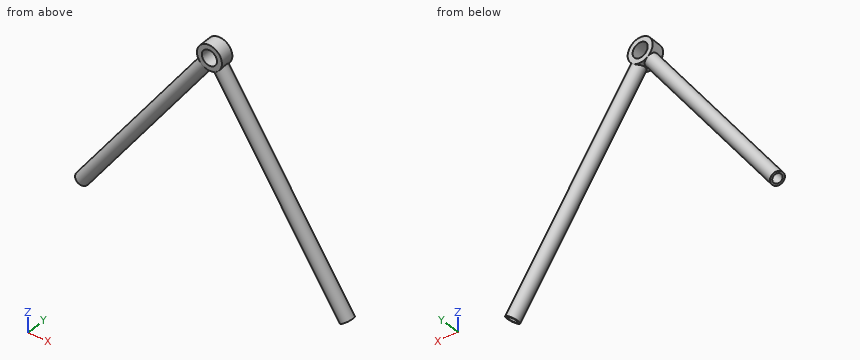
from build123d import *

# Parameters (mm, degrees)
SKETCH1_R                = 19.0062
SKETCH1_R_2              = 11.5062
BOSS_EXTRUDE1_DEPTH      = 10
BOSS_EXTRUDE2_REACH      = 392.082
BOSS_EXTRUDE2_END_RADIUS = 19.0062
SKETCH5_R                = 10
SKETCH5_R_2              = 7
BOSS_EXTRUDE3_REACH      = 510.057
BOSS_EXTRUDE3_END_RADIUS = 19.0062
SKETCH6_R                = 10
SKETCH6_R_2              = 7


with BuildPart() as part:
    # Sketch1 → Boss-Extrude1 (new, symmetric)
    with BuildSketch(Plane(origin=(0, 0, 0), x_dir=(1, 0, 0), z_dir=(0, 1, 0))):
        with Locations(Location((0, 0, 0), (0, 0, 270))):
            Circle(SKETCH1_R)
        with Locations(Location((0, 0, 0), (0, 0, 270))):
            Circle(SKETCH1_R_2, mode=Mode.SUBTRACT)
    extrude(amount=BOSS_EXTRUDE1_DEPTH, both=True)

    # Boss-Extrude2: up to this cylinder (the profile starts outside it)
    boss_extrude2_end = Plane(origin=(0, 0, 0), z_dir=(0, -1, 0)) * Cylinder(BOSS_EXTRUDE2_END_RADIUS, 823.1764, mode=Mode.PRIVATE)
    # Sketch5 → Boss-Extrude2 (add, up to the surface)
    with BuildSketch(Plane(origin=(201.884851726, 0, -302.352155823), x_dir=(0.8316479627965052, 0, 0.555303219850581), z_dir=(0.555303219850581, 0, -0.8316479627965052)), mode=Mode.PRIVATE) as boss_extrude2_sk1:
        with Locations(Location((0, 0, 0), (0, 0, 180))):
            Circle(SKETCH5_R)
        with Locations(Location((0, 0, 0), (0, 0, 180))):
            Circle(SKETCH5_R_2, mode=Mode.SUBTRACT)
    boss_extrude2_tool1 = extrude(boss_extrude2_sk1.sketch, amount=-BOSS_EXTRUDE2_REACH, mode=Mode.PRIVATE) - boss_extrude2_end
    add(boss_extrude2_tool1.solids().sort_by_distance((209.966106, 0, -296.956187))[0])

    # Boss-Extrude3: up to this cylinder (the profile starts outside it)
    boss_extrude3_end = Plane(origin=(0, 0, 0), z_dir=(0, -1, 0)) * Cylinder(BOSS_EXTRUDE3_END_RADIUS, 1059.1264, mode=Mode.PRIVATE)
    # Sketch6 → Boss-Extrude3 (add, up to the surface)
    with BuildSketch(Plane(origin=(-200.97050419, 0, -279.254437795), x_dir=(-0.811662071535183, 0, 0.5841272820466578), z_dir=(-0.5841272820466578, 0, -0.811662071535183)), mode=Mode.PRIVATE) as boss_extrude3_sk1:
        Circle(SKETCH6_R)
        Circle(SKETCH6_R_2, mode=Mode.SUBTRACT)
    boss_extrude3_tool1 = extrude(boss_extrude3_sk1.sketch, amount=-BOSS_EXTRUDE3_REACH, mode=Mode.PRIVATE) - boss_extrude3_end
    add(boss_extrude3_tool1.solids().sort_by_distance((-193.083456, 0, -284.930494))[0])


solid = part.part
For this review, take the finished solid that the model builds, in its own axes (mm). Give positions to 0.01 mm unless a question says otherwise; leave off trailing zeros. Order: outer loops, then holes, each group sorted by start corner. A loop starts at its lowest first (then second) coordinate and runs counter-clockwise, first axis right, second up. Notation, with made-up numbers: (-6, 7.25) -> (44, 7.25) arc R8 cw to (44, 12.25) -> close; hole circle Ø3 at (77, 61). An arc over 180 degrees is marked (long way). Write item = value, one per line.
1) We need section B-B, the plane y = 3.25. Give the boundary of the cut face in (x, z), and give its area (3 significant figures).
Findings:
outline = (-208.65, -273.73) -> (-206, -275.63) -> (-15.53, -10.96) arc R19.01 ccw to (-5.46, -18.2) -> (-195.94, -282.88) -> (-193.29, -284.78) -> (-1.95, -18.91) arc R19.01 ccw to (1.29, -18.96) -> (194.02, -307.6) -> (196.73, -305.79) -> (4.82, -18.38) arc R19.01 ccw to (15.13, -11.5) -> (207.04, -298.91) -> (209.75, -297.1) -> (17.02, -8.46) arc R19.01 ccw (long way) to (-17.31, -7.86) -> close; hole circle Ø23.01 at (0, 0)
area = 5,100 mm^2
2) We need section A-A, the plane z = 0. Give the boundary of the cut face in (x, y), and give its area (3 significant figures).
Findings:
outline = (-19.01, -10) -> (-11.51, -10) -> (-11.51, 10) -> (-19.01, 10) -> close; (11.51, -10) -> (19.01, -10) -> (19.01, 10) -> (11.51, 10) -> close
area = 300 mm^2
3) To check wall thickness, follow L1, parallel to X at y = 4.5, z = 0; L2, parallel to Y at x = 35.5, z = -52.5; L3, parallel to X at y = 1, z = -129. State the ranges of each line that lie inside material, in increasing order. Write a range as from..to.
Findings:
L1 = -19.01..-11.51, 11.51..19.01
L2 = -9.99..-6.99, 6.99..9.99
L3 = -105.1..-101.37, -84.3..-80.58, 74.17..77.8, 94.47..98.1
4) We need section C-C, the plane z = -117.5. Count the separate pieces of the cut face and the enclosed holes in it, and give its area (3 significant figures).
Findings:
separate_pieces = 2
enclosed_holes = 2
area = 390 mm^2
5) Insertion check: pin 1 (1.5 mm diameter, centred on x = -16.5, y = -1, fed in from +Z); pin 2 (12 mm diameter, centred on y = 7.5, z = -161.5, fed in from +X); pin 3 (10 mm diameter, centred on x = -33.5, z = -62.5, fed in from -Y). Each pin has a flat end and moves straight along its axis. Give the tip position at first contact, or say it passes through.
Findings:
pin_1 = 10.64
pin_2 = 122.11
pin_3 = -9.02
